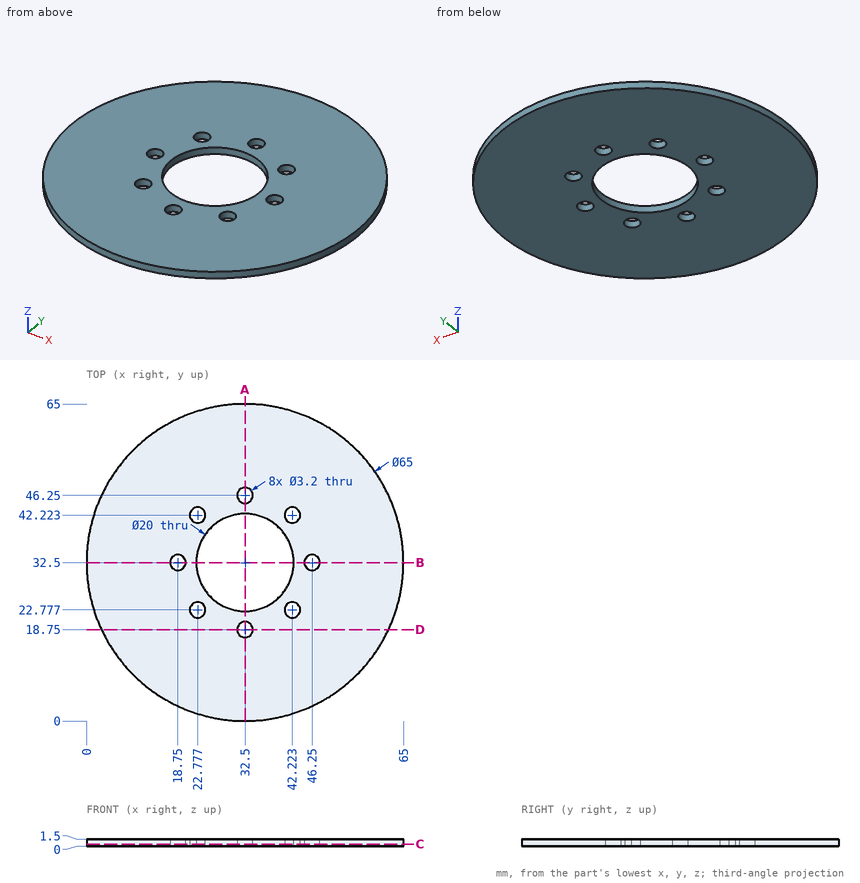
Here's the drawing with two shaded views (mm, measured from the low corner). I have some questions. Round coordinates to 2 decimals unless told otherwise and drop trailing zeros. Write each loop counter-clockwise with the first axis right and the second up, starting at its lowest first coordinate (ties: lowest second). Pieces come first, ordered by that corner, then holes.
(1) Suppose I cut it at C-C on z = 0.45. State how many separate pieces and enclosed holes the cut face has, and give its area (3 significant figures).
Findings below:
separate pieces: 1
enclosed holes: 9
area: 2,940 mm2
(2) If I drill on probe 1 along Y at (x, z) = (32.5, 1); probe 2 along Y at (x, z) = (43.5, 1.45) (1 decimal); probe 3 along Y at (x, z) = (40, 0.6) (1 decimal), over which ranges is the centre line in solid material (lowest first)?
Findings below:
probe 1: y = 0 to 17.15, 20.35 to 22.5, 42.5 to 44.65, 47.85 to 65
probe 2: y = 1.9 to 21.8, 23.7 to 41.3, 43.2 to 63.1
probe 3: y = 0.9 to 25.9, 39.1 to 64.1
(3) Suppose I cut it at A-A on x = 32.5. Write out the boundary of the cut face in (y, z).
Findings below:
outline: (0, 0) - (17.15, 0) - (17.15, 1.5) - (0, 1.5) - close; (20.35, 0) - (22.5, 0) - (22.5, 1.5) - (20.35, 1.5) - close; (42.5, 0) - (44.65, 0) - (44.65, 1.5) - (42.5, 1.5) - close; (47.85, 0) - (65, 0) - (65, 1.5) - (47.85, 1.5) - close
(4) Suppose I cut it at D-D on y = 18.75. Write out the boundary of the cut face in (x, z).
Findings below:
outline: (3.05, 0) - (30.9, 0) - (30.9, 1.5) - (3.05, 1.5) - close; (34.1, 0) - (61.95, 0) - (61.95, 1.5) - (34.1, 1.5) - close
(5) For pin 1 (3.5 mm diameter, centred on x = 22.78, y = 42.22, fed in from +Z), with a flat end and sliding along its axis, tell me the tip position at first contact or that it passes through.
Findings below:
pin 1: stops at z = 1.5
